Geometry check sheet. Reference: the model listing, model coordinates, mm. A direction names the side the tool comes from. Give positions to 0.01 mm unless a question says otherwise; leave off trailing zeros. Write each loop counter-clockwise with the first axis right and the second up, starting at its lowest first coordinate (ties: lowest second). Pieces come first, ordered by that corner, then holes. Notation, with made-up numbers: M -34,-30 L 1,-30 A30 ccw 1,-4 Z; hole C 7.5,63.5 d1. An arc over 180 degrees is marked long. One line per item, written item: value. Start each with the question number.
1. Gauge pin test, flat ends, axial feed: pin 1 (3.5 mm diameter, centred on x = 19, y = 2, fed in from -Z); pin 2 (6 mm diameter, centred on y = 4.5, z = 15, fed in from +X); pin 3 (2 mm diameter, centred on y = 2.5, z = -0.5, fed in from +X); pin 4 (1.8 mm diameter, centred on x = 0, z = -6.5, fed in from -Y). Record the tip position at first contact, or that the pin passes through.
2. Cross-section at A-A on x = 11. Record the cut outline in (y, z), then the cut area to 3 significant figures.
3. Cross-section at C-C on x = 19. Record the cut outline in (y, z).
4. Cross-section at D-D on y = 19.73. Record the cut outline in (x, z), then the cut area to 3 significant figures.
5. Tool access check on faces 4 (the face through (20, 16, -7)), 5 (the face through (0, 1.1, 2)), 6 (the face through (13, 4, -4)), 7 (the face through (0.044, 0.542, 16.875)). Record the directions out of +Z, -Z, +X, -X, +Y, -Y that give a thin tool (end or side, any length) a straight path to the whole face; none if there is none.
6. Release check for a two-part mould opening along Y. For faces 1 (the face through (0, 4, -13.75)), 2 (the face through (20.43, 9.24, -0.55)), 3 (the face through (8, 0, 5)) record: pulls with the +Y half, pulls with the -Y half, needs draft (parallel to the pull), parting line crosses it, or undercut.
7. Scan lines: line 1 (Y direction, x = 20, z = 0); line 2 (X direction, y = 5.5, z = 6.5); line 3 (Y direction, x = 0.5, z = 15.5). Record each from-to range of solid material in increasing order.
8. Cross-section at B-B on y = 3.73. Record the cut outline in (x, z), then the cut area to 3 significant figures.
from build123d import *

# Parameters (mm, degrees)
SKETCH1_W           = 8.2
SKETCH1_H           = 8
BOSS_EXTRUDE1_DEPTH = 7.46
BOSS_EXTRUDE2_DEPTH = 16.34
SKETCH4_R           = 2.55
CUT_EXTRUDE1_DEPTH  = 43.142763317
CUT_EXTRUDE2_DEPTH  = 1.1
CUT_EXTRUDE4_REACH  = 42.752
SKETCH6_R           = 1


with BuildPart() as part:
    # Sketch1 → Boss-Extrude1 (new body)
    with BuildSketch(Plane(origin=(0, 0, 0), x_dir=(1, 0, 0), z_dir=(0, 1, 0))):
        Polygon((8.75, 11.46), (24.21, 11.46), (24.21, -11.46), (8.75, -11.46), (8.75, -23.65), (-8.75, -23.65), (-8.75, 13.75), (8.75, 13.75), align=None)
        with Locations((12.65, 0)):
            Rectangle(SKETCH1_W, SKETCH1_H, mode=Mode.SUBTRACT)
    extrude(amount=BOSS_EXTRUDE1_DEPTH)

    # Sketch3 → Boss-Extrude2 (add)
    with BuildSketch(Plane(origin=(0, 7.46, 0), x_dir=(1, 0, 0), z_dir=(0, 1, 0))):
        Polygon((16.75, 7), (24.21, 7), (24.21, -7), (16.75, -7), (16.75, -4), (16.75, 4), align=None)
    extrude(amount=BOSS_EXTRUDE2_DEPTH)

    # Sketch4 → Cut-Extrude1 (cut, through all)
    with BuildSketch(Plane.ZY.offset(-16.75)):
        with Locations((0, 3.73)):
            Circle(SKETCH4_R)
        with Locations((0, 11.73)):
            Circle(SKETCH4_R)
        with Locations((0, 19.73)):
            Circle(SKETCH4_R)
    extrude(amount=-CUT_EXTRUDE1_DEPTH, mode=Mode.SUBTRACT)

    # Sketch5 → Cut-Extrude2 (cut)
    with BuildSketch(Plane.XZ):
        with BuildLine():
            Line((-2.113983221, 14.966101695), (-3.606206671, 0.368644068))
            ThreePointArc((-3.606206671, 0.368644068), (-3.625, 0), (-3.606206671, -0.368644068))
            Line((-3.606206671, -0.368644068), (-2.113983221, -14.966101695))
            ThreePointArc((-2.113983221, -14.966101695), (0, -16.875), (2.113983221, -14.966101695))
            Line((2.113983221, -14.966101695), (3.606206671, -0.368644068))
            ThreePointArc((3.606206671, -0.368644068), (3.625, 0), (3.606206671, 0.368644068))
            Line((3.606206671, 0.368644068), (2.113983221, 14.966101695))
            ThreePointArc((2.113983221, 14.966101695), (0, 16.875), (-2.113983221, 14.966101695))
        make_face()
    extrude(amount=-CUT_EXTRUDE2_DEPTH, mode=Mode.SUBTRACT)

    # Sketch6 → Cut-Extrude4 (cut, up to next)
    with BuildSketch(Plane.XZ.offset(-1.1), mode=Mode.PRIVATE) as cut_extrude4_sk1:
        with Locations(Location((0, 12.6, 0), (0, 0, 270))):
            Circle(SKETCH6_R)
    cut_extrude4_tool1 = extrude(cut_extrude4_sk1.sketch, amount=-CUT_EXTRUDE4_REACH, mode=Mode.PRIVATE) & part.part
    # Sketch6 → Cut-Extrude4 (cut, up to next)
    with BuildSketch(Plane.XZ.offset(-1.1), mode=Mode.PRIVATE) as cut_extrude4_sk2:
        with Locations(Location((0, 6.5, 0), (0, 0, 270))):
            Circle(SKETCH6_R)
    cut_extrude4_tool2 = extrude(cut_extrude4_sk2.sketch, amount=-CUT_EXTRUDE4_REACH, mode=Mode.PRIVATE) & part.part
    # Sketch6 → Cut-Extrude4 (cut, up to next)
    with BuildSketch(Plane.XZ.offset(-1.1), mode=Mode.PRIVATE) as cut_extrude4_sk3:
        with Locations(Location((0, -6.5, 0), (0, 0, 270))):
            Circle(SKETCH6_R)
    cut_extrude4_tool3 = extrude(cut_extrude4_sk3.sketch, amount=-CUT_EXTRUDE4_REACH, mode=Mode.PRIVATE) & part.part
    add(cut_extrude4_tool1.solids().sort_by_distance((0, 1.1, 12.6))[0], mode=Mode.SUBTRACT)
    add(cut_extrude4_tool2.solids().sort_by_distance((0, 1.1, 6.5))[0], mode=Mode.SUBTRACT)
    add(cut_extrude4_tool3.solids().sort_by_distance((0, 1.1, -6.5))[0], mode=Mode.SUBTRACT)


solid = part.part
Report:
1. pin 1: stops at z = -11.46
1. pin 2: stops at x = 8.75
1. pin 3: stops at x = 8.55
1. pin 4: passes through
2. outline: M 0,-11.46 L 7.46,-11.46 L 7.46,-4 L 0,-4 Z; M 0,4 L 7.46,4 L 7.46,11.46 L 0,11.46 Z
2. area: 111 mm^2
3. outline: M 0,-11.46 L 7.46,-11.46 L 7.46,-7 L 23.8,-7 L 23.8,7 L 7.46,7 L 7.46,11.46 L 0,11.46 Z; hole C 3.73,0 d5.1; hole C 11.73,0 d5.1; hole C 19.73,0 d5.1
4. outline: M 16.75,-7 L 24.21,-7 L 24.21,-2.55 L 16.75,-2.55 Z; M 16.75,2.55 L 24.21,2.55 L 24.21,7 L 16.75,7 Z
4. area: 66.4 mm^2
5. face 4: -Z, +X, -X, +Y
5. face 5: -Y
5. face 6: +Y, -Y
5. face 7: -Z, -Y
6. face 1: needs draft
6. face 2: undercut
6. face 3: pulls with the -Y half
7. line 1: y = 0 to 1.18, 6.28 to 9.18, 14.28 to 17.18, 22.28 to 23.8
7. line 2: x = -8.75 to -1, 1 to 24.21
7. line 3: y = 1.1 to 7.46
8. outline: M -8.75,-13.75 L 8.75,-13.75 L 8.75,-11.46 L 24.21,-11.46 L 24.21,-2.55 L 16.75,-2.55 L 16.75,-4 L 8.55,-4 L 8.55,4 L 16.75,4 L 16.75,2.55 L 24.21,2.55 L 24.21,11.46 L 8.75,11.46 L 8.75,23.65 L -8.75,23.65 Z; hole C 0,-6.5 d2; hole C 0,6.5 d2; hole C 0,12.6 d2
8. area: 896 mm^2
